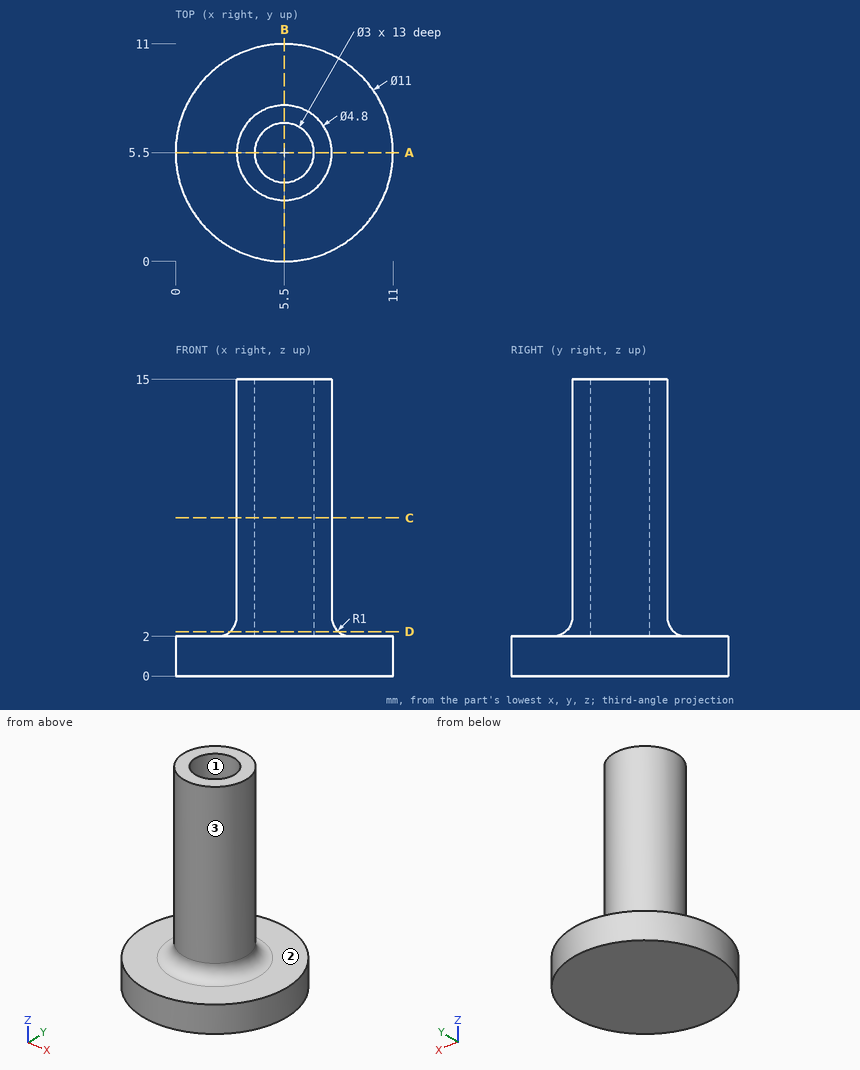
Input: dimensioned drawing with shaded views. Units: mm. Origin: part minimum x, y, z. Round coordinates to 2 decimals unless told otherwise and drop trailing zeros. Order: outer loops, then holes, each group sorted by start corner. A loop starts at its lowest first (then second) coordinate and runs counter-clockwise, first axis right, second up. Notation, with made-up numbers: M 84.5,-16.75 L 136.5,-16.75 A12 cw 136.5,-2.75 Z; hole C 18,73 d7. An arc over 180 degrees is marked long. Use one line per item in the form item = value. Start each with the question number.
Q1. Pin query (flat end, axial travel): pin 1 Ø1 at (x, z) = (6.5, 12.5) entering from -Y; pin 2 Ø1.5 at (y, z) = (5, 11.5) entering from -X; pin 3 Ø3 at (y, z) = (6, 9) entering from +X; pin 4 Ø3.5 at (x, y) = (5.5, 5.5) entering from +Z. Return the tip coordinate at first contact, or that it passes through.
Q2. Cut plane C-C (z = 8). Return loops of the section in (x, y).
Q3. Material intervals for line 1 (X direction, y = 5.5, z = 9.75); line 2 (Z direction, x = 6.5, y = 6), sorted ascending. Write a range as [from, to].
Q4. Cut plane D-D (z = 2.25). Return loops of the section in (x, y).
Q5. Mould query, pull axis X, two halves, no side actions, for the marked faces 1, 2 and 3. Classes: +X half, -X half, draft (parallel to the pull), parting line (faces both ways), or undercut.
Q6. Cut plane A-A (y = 5.5). Return loops of the section in (x, z).
Geometry results:
q1.pin_1 = 3.15
q1.pin_2 = 3.1
q1.pin_3 = 7.9
q1.pin_4 = 15
q2.outline = C 5.5,5.5 d4.8; hole C 5.5,5.5 d3
q3.line_1 = [3.1, 4], [7, 7.9]
q3.line_2 = [0, 2]
q4.outline = C 5.5,5.5 d5.48; hole C 5.5,5.5 d3
q5.face_1 = undercut
q5.face_2 = draft
q5.face_3 = parting line
q6.outline = M 0,0 L 11,0 L 11,2 L 8.9,2 A1 cw 7.9,3 L 7.9,15 L 7,15 L 7,2 L 4,2 L 4,15 L 3.1,15 L 3.1,3 A1 cw 2.1,2 L 0,2 Z
